Can you work these out from the model? Positions are in its coordinate system, mm. Round coordinates to 2 decimals unless told otherwise and drop trailing zeros. Order: outer loops, then holes, each group sorted by start corner. A loop starts at its lowest first (then second) coordinate and runs counter-clockwise, first axis right, second up.
from build123d import *

# Parameters (mm, degrees)
CROQUIS1_R              = 4.5
SALIENTE_EXTRUIR1_DEPTH = 28.32
REDONDEO1_R             = 10


with BuildPart() as part:
    # Croquis1 → Saliente-Extruir1 (new body)
    with BuildSketch(Plane.XY):
        Polygon((14.527798388, -0.008569378), (38.527798388, -0.032811814), (38.527798388, -5.044933007), (38.527798388, -30.044933007), (14.527798388, -30.044933007), (14.527798388, -5.044933007), align=None)
        with Locations((26.527798388, -17.544933007)):
            Circle(CROQUIS1_R, mode=Mode.SUBTRACT)
    extrude(amount=SALIENTE_EXTRUIR1_DEPTH)

    # Redondeo1
    redondeo1_edges = [part.edges().sort_by_distance(p)[0] for p in [
        (14.527798388, -30.044933007, 14.16),
        (38.527798388, -30.044933007, 14.16),
    ]]
    fillet(redondeo1_edges, radius=REDONDEO1_R)


solid = part.part
(1) Please list where these lines run through material, in increasing order: probe 1 along Y at (x, z) = (22.75, 25); probe 2 along X at (y, z) = (-18.5, 12); probe 3 along X at (y, z) = (-21.5, 11.75).
(2) I want a section at D-D, the plane x = 20.25. List the corners of the cut face in (y, z) for me.
(3) I want a section at A-A, the plane x = 29. List the corners of the cut face in (y, z) for me, plus the area to 3 significant figures.
(4) I want a section at C-C, the plane z = 17. List the corners of the cut face in (x, y) for me, plus the area to 3 significant figures.
(5) If we mould it in two halves opening along X, with no side actions, what happens to faces 1 (the face through (17.38, -27.04, 14.36)), 2 (the face through (30.82, -16.19, 13.96)), 3 (the face through (27, -11, 28.32))? For each: pulls with the +X half, pulls with the -X half, needs draft (parallel to the pull), parting line crosses it, or undercut.
(6) I want a section at B-B, the plane y = -17. List the corners of the cut face in (x, z) for me.
(7) I'm going to push flat-ended pins straight in: pin 1 Ø7 at (x, y) = (26.53, -17.54) entering from -Z; pin 2 Ø12 at (x, z) = (26.5, 16.5) entering from +Y; pin 3 Ø3 at (x, z) = (22, 24.5) entering from -Y; pin 4 Ø2 at (x, z) = (35, 7.5) entering from -Y. Where does each tip first touch, or does it pass through?
Ans:
1. probe 1: y = -29.89 to -19.99, -15.1 to -0.02
1. probe 2: x = 14.53 to 22.13, 30.93 to 38.53
1. probe 3: x = 14.63 to 24.38, 28.67 to 38.42
2. outline: (-29.08, 0) - (-0.01, 0) - (-0.01, 28.32) - (-29.08, 28.32) - close
3. outline: (-30.03, 0) - (-21.31, 0) - (-21.31, 28.32) - (-30.03, 28.32) - close; (-13.78, 0) - (-0.02, 0) - (-0.02, 28.32) - (-13.78, 28.32) - close
3. area: 637 mm2
4. outline: (14.53, -20.04) arc R10 ccw to (24.53, -30.04) - (28.53, -30.04) arc R10 ccw to (38.53, -20.04) - (38.53, -0.03) - (14.53, -0.01) - close; hole circle Ø9 at (26.53, -17.54)
4. area: 614 mm2
5. face 1: pulls with the -X half
5. face 2: undercut
5. face 3: needs draft
6. outline: (14.53, 0) - (22.06, 0) - (22.06, 28.32) - (14.53, 28.32) - close; (30.99, 0) - (38.53, 0) - (38.53, 28.32) - (30.99, 28.32) - close
7. pin 1: passes through
7. pin 2: stops at y = -0.01
7. pin 3: stops at y = -29.99
7. pin 4: stops at y = -28.41
